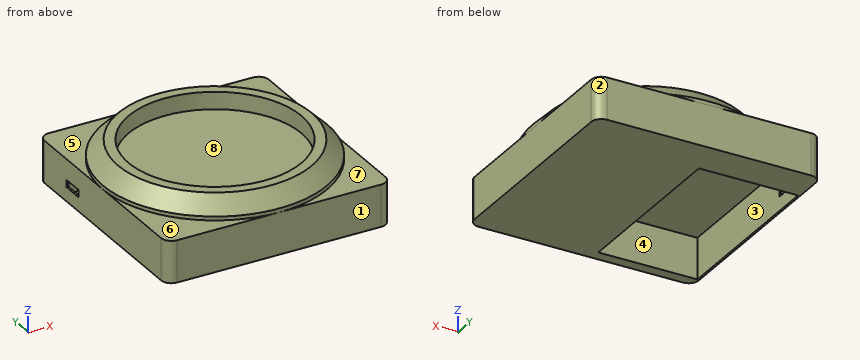
from build123d import *

# Parameters (mm, degrees)
F0_R      = 55.499
F0_R_2    = 42.799
F1_DEPTH  = 9.525
F2_W      = 110.998
F2_H      = 110.998
F3_DEPTH  = 20.701
F4_SIZE   = 7.62
F5_W      = 49.022
F5_H      = 87.122
F6_DEPTH  = 20.32
F7_W      = 10.16
F7_H      = 3.556
F8_DEPTH  = 1
F9_R      = 5
F10_R     = 42.799
F11_DEPTH = 1


with BuildPart() as f1:
    # F0 (on Top) → F1 (new body)
    with BuildSketch(Plane.XY):
        Circle(F0_R)
        Circle(F0_R_2, mode=Mode.SUBTRACT)
    extrude(amount=F1_DEPTH)

    # F2 (on face) → F3 (join)
    with BuildSketch(Plane(origin=(0, 0, 0), x_dir=(1, 0, 0), z_dir=(0, 0, -1))):
        Rectangle(F2_W, F2_H)
    extrude(amount=F3_DEPTH)

    # F4
    f4_edges = [f1.edges().sort_by_distance(p)[0] for p in [
        (-55.499, 0, 9.525),
    ]]
    chamfer(f4_edges, length=F4_SIZE)

    # F5 (on face) → F6 (cut)
    with BuildSketch(Plane(origin=(0, 0, -20.701), x_dir=(1, 0, 0), z_dir=(0, 0, -1))):
        with Locations((-29.988, 6.413653)):
            Rectangle(F5_W, F5_H)
    extrude(amount=-F6_DEPTH, mode=Mode.SUBTRACT)

    # F7 (on face) → F8 (cut, through all)
    with BuildSketch(Plane(origin=(-55.499, 0, 0), x_dir=(0, -1, 0), z_dir=(-1, 0, 0))):
        with Locations((-26.352347, -11.938)):
            Rectangle(F7_W, F7_H)
    extrude(amount=-F8_DEPTH, mode=Mode.SUBTRACT)

    # F9
    f9_edges = [f1.edges().sort_by_distance(p)[0] for p in [
        (-55.499, -55.499, -10.3505),
        (-55.499, 55.499, -10.3505),
        (55.499, -55.499, -10.3505),
        (55.499, 55.499, -10.3505),
    ]]
    fillet(f9_edges, radius=F9_R)

    # F10 (on face) → F11 (join)
    with BuildSketch(Plane.XY):
        Circle(F10_R)
    extrude(amount=F11_DEPTH)


solid = f1.part
The listing builds one solid part. Answer for the finished solid, in the listing's coordinates (mm). Face numbers are marked on the shaded views. A direction names the side the tool comes from. Round coordinates to 2 decimals unless told otherwise and drop trailing zeros. Loops run counter-clockwise (first coordinate to the right, second up) from the corner with the lowest first, then second, coordinate; pieces in that order, holes last. Notation, with made-up numbers: M 45.25,46 L 84.25,46 A37 cw 84.25,83 Z; hole C 58.25,63.25 d6. An arc over 180 degrees is marked long. Return JSON: item names as keys, results as strings.
Q1. Each of these flat-tipped pins is pushed along its axis until it touches: pin 1 Ø0.8 at (x, z) = (-55, -12) entering from -Y; pin 2 Ø0.5 at (x, y) = (-55, 24.5) entering from +Z; pin 3 Ø1.5 at (x, y) = (-28.5, 9.5) entering from +Z; pin 4 Ø2 at (x, z) = (15.5, 0.5) entering from -Y. Where does it stop, or does it pass through?
Results list:
{"pin 1": "stops at y = -53.36", "pin 2": "stops at z = 0", "pin 3": "stops at z = 1", "pin 4": "stops at y = -55.5"}
Q2. Find the intervals of material crossed by line 1 along X through (y, z) = (-35, -5); line 2 along Z through (x, y) = (1.5, 1.5); line 3 along Z through (x, y) = (-10.5, 3.5), in increasing order. Write a range as from..to.
Results list:
{"line 1": "x = -55.5..-54.5, -5.48..55.5", "line 2": "z = -20.7..1", "line 3": "z = -0.38..1"}
Q3. The mould has two halves that part along X. Classify the marked faces 1, 2 and 3: released by +X, released by -X, zero draft, split by the parting line, or undercut.
Results list:
{"face 1": "zero draft", "face 2": "released by +X", "face 3": "undercut"}
Q4. Find section A-A, the plane z = -16. Determine the outline of the cut face in (x, y), plus the area to 3 significant figures.
Results list:
{"outline": "M -55.5,-50.5 A5 ccw -50.5,-55.5 L 50.5,-55.5 A5 ccw 55.5,-50.5 L 55.5,50.5 A5 ccw 50.5,55.5 L -50.5,55.5 A5 ccw -55.5,50.5 Z; hole M -54.5,-49.97 L -5.48,-49.97 L -5.48,37.15 L -54.5,37.15 Z", "area": "8,030 mm2"}
Q5. Which of the six approach directions +Z, -Z, +X, -X, +Y, -Y give full straight-line access (tool end or side, diameter ignored) to the marked faces 4, 5, 6, 7 and 8?
Results list:
{"face 4": "-Z", "face 5": "+Z, -X, +Y", "face 6": "+Z, -X, -Y", "face 7": "+Z, +X, -Y", "face 8": "+Z"}
